```python
from build123d import *

# Parameters (mm, degrees)
SKETCH2_W           = 40.5
SKETCH2_H           = 41
BOSS_EXTRUDE1_DEPTH = 20
SKETCH4_W           = 20
SKETCH4_H           = 4
BOSS_EXTRUDE2_DEPTH = 7.95
SKETCH5_W           = 20
SKETCH5_H           = 4
BOSS_EXTRUDE3_DEPTH = 7.95
SKETCH8_R           = 2.5
CUT_EXTRUDE1_DEPTH  = 45.488650238
SKETCH11_R          = 3.792509707
BOSS_EXTRUDE4_DEPTH = 7


with BuildPart() as part:
    # Sketch2 → Boss-Extrude1 (new body)
    with BuildSketch(Plane.XY):
        Rectangle(SKETCH2_W, SKETCH2_H)
    extrude(amount=BOSS_EXTRUDE1_DEPTH)

    # Sketch4 → Boss-Extrude2 (add)
    with BuildSketch(Plane(origin=(20.25, 0, 0), x_dir=(0, 0, -1), z_dir=(1, 0, 0))):
        with Locations((-10, 5.5)):
            Rectangle(SKETCH4_W, SKETCH4_H)
    extrude(amount=BOSS_EXTRUDE2_DEPTH)

    # Sketch5 → Boss-Extrude3 (add)
    with BuildSketch(Plane.ZY.offset(20.25)):
        with Locations((10, 5.5)):
            Rectangle(SKETCH5_W, SKETCH5_H)
    extrude(amount=BOSS_EXTRUDE3_DEPTH)

    # Sketch8 → Cut-Extrude1 (cut, through all)
    with BuildSketch(Plane(origin=(0, 7.5, 0), x_dir=(1, 0, 0), z_dir=(0, 1, 0))):
        with Locations(Location((24, -5, 0), (0, 0, 270))):
            Circle(SKETCH8_R)
        with Locations(Location((24, -15, 0), (0, 0, 270))):
            Circle(SKETCH8_R)
        with Locations(Location((-24, -5, 0), (0, 0, 270))):
            Circle(SKETCH8_R)
        with Locations(Location((-24, -15, 0), (0, 0, 270))):
            Circle(SKETCH8_R)
    extrude(amount=-CUT_EXTRUDE1_DEPTH, mode=Mode.SUBTRACT)

    # Sketch11 → Boss-Extrude4 (add)
    with BuildSketch(Plane(origin=(0, 20.5, 0), x_dir=(1, 0, 0), z_dir=(0, 1, 0))):
        with Locations(Location((10.25, -10, 0), (0, 0, 90))):
            Circle(SKETCH11_R)
    extrude(amount=BOSS_EXTRUDE4_DEPTH)


solid = part.part
```
Work out the finished part from the listing and answer in its coordinate system (mm). A direction names the side the tool comes from. Round coordinates to 2 decimals unless told otherwise and drop trailing zeros. Write each loop counter-clockwise with the first axis right and the second up, starting at its lowest first coordinate (ties: lowest second). Pieces come first, ordered by that corner, then holes. Notation, with made-up numbers: (14, 17.25) -> (36, 17.25) arc R5 ccw to (36, 25.25) -> close; hole circle Ø3 at (50.25, 74.5). An arc over 180 degrees is marked (long way). Write each question's results on one line, items separated by ' | '.
1) The part is cut by section C-C (x = 10.25). Write down the section's boundary in (y, z).
Findings:
outline: (-20.5, 0) -> (20.5, 0) -> (20.5, 6.21) -> (27.5, 6.21) -> (27.5, 13.79) -> (20.5, 13.79) -> (20.5, 20) -> (-20.5, 20) -> close
2) Flat-ended cylindrical pins translate along their axes: pin 1 (6.5 mm diameter, centred on y = 12.5, z = 8, fed in from +X); pin 2 (6 mm diameter, centred on y = -13.5, z = 14, fed in from -X); pin 3 (6.5 mm diameter, centred on x = -24, z = 10.5, fed in from -Y). Find the tip coordinate at first contact, or state that the pin passes through.
Findings:
pin 1: stops at x = 20.25 | pin 2: stops at x = -20.25 | pin 3: stops at y = 3.5
3) Which of the six approach directions +Z, -Z, +X, -X, +Y, -Y give full straight-line access (tool end or side, diameter ignored) to faces 1 (the flat face through (20.25, -9, 10)), 2 (the flat face through (-24, 7.5, 10)), 3 (the flat face through (24, 7.5, 10))?
Findings:
face 1: +Z, -Z, +X, -Y | face 2: +Z, -Z, -X, +Y | face 3: +Z, -Z, +X, +Y
4) The part is cut by section D-D (z = 15). Write down the section's boundary in (x, y), and give its area (3 significant figures).
Findings:
outline: (-28.2, 3.5) -> (-26.5, 3.5) -> (-26.5, 7.5) -> (-28.2, 7.5) -> close; (-21.5, 3.5) -> (-20.25, 3.5) -> (-20.25, -20.5) -> (20.25, -20.5) -> (20.25, 3.5) -> (21.5, 3.5) -> (21.5, 7.5) -> (20.25, 7.5) -> (20.25, 20.5) -> (-20.25, 20.5) -> (-20.25, 7.5) -> (-21.5, 7.5) -> close; (26.5, 3.5) -> (28.2, 3.5) -> (28.2, 7.5) -> (26.5, 7.5) -> close | area: 1,680 mm²
5) The part is cut by section A-A (z = 3.5). Write down the section's boundary in (x, y).
Findings:
outline: (-28.2, 3.5) -> (-26, 3.5) -> (-26, 7.5) -> (-28.2, 7.5) -> close; (-22, 3.5) -> (-20.25, 3.5) -> (-20.25, -20.5) -> (20.25, -20.5) -> (20.25, 3.5) -> (22, 3.5) -> (22, 7.5) -> (20.25, 7.5) -> (20.25, 20.5) -> (-20.25, 20.5) -> (-20.25, 7.5) -> (-22, 7.5) -> close; (26, 3.5) -> (28.2, 3.5) -> (28.2, 7.5) -> (26, 7.5) -> close
6) The part is cut by section B-B (x = -24). Write down the section's boundary in (y, z), and give its area (3 significant figures).
Findings:
outline: (3.5, 0) -> (7.5, 0) -> (7.5, 2.5) -> (3.5, 2.5) -> close; (3.5, 7.5) -> (7.5, 7.5) -> (7.5, 12.5) -> (3.5, 12.5) -> close; (3.5, 17.5) -> (7.5, 17.5) -> (7.5, 20) -> (3.5, 20) -> close | area: 40.0 mm²
7) For a pull along Z with two mould halves and no side action, classify faces 4 (the cylindrical face through (-22.31, 5.53, 13.16)), 5 (the flat face through (0, 0, 0)), 6 (the flat face through (-20.25, -9, 10)) as +Z half, -Z half, draft (parallel to the pull), parting line (faces both ways), or undercut.
Findings:
face 4: undercut | face 5: -Z half | face 6: draft
8) Consider line 1 along X through (y, z) = (5.9, 15); line 2 along X through (y, z) = (4.5, 6); line 3 along Y through (x, z) = (-14, 11.5). Determine where each line is inside the solid, lowest interval first. Write a range as [from, to].
Findings:
line 1: x = [-28.2, -26.5], [-21.5, 21.5], [26.5, 28.2] | line 2: x = [-28.2, -26.29], [-21.71, 21.71], [26.29, 28.2] | line 3: y = [-20.5, 20.5]
